For this review, take the finished solid that the model builds, in its own axes (mm). Face numbers are marked on the shaded views. A direction names the side the tool comes from. Round coordinates to 2 decimals unless told otherwise and drop trailing zeros. Order: outer loops, then holes, each group sorted by start corner. A loop starts at its lowest first (then second) coordinate and runs counter-clockwise, first axis right, second up. Notation, with made-up numbers: M 72.5,35.5 L 96.5,35.5 A26 ccw 96.5,62.5 Z; hole C 65.25,75 d5. An arc over 180 degrees is marked long. Use a Markdown table: item, result.
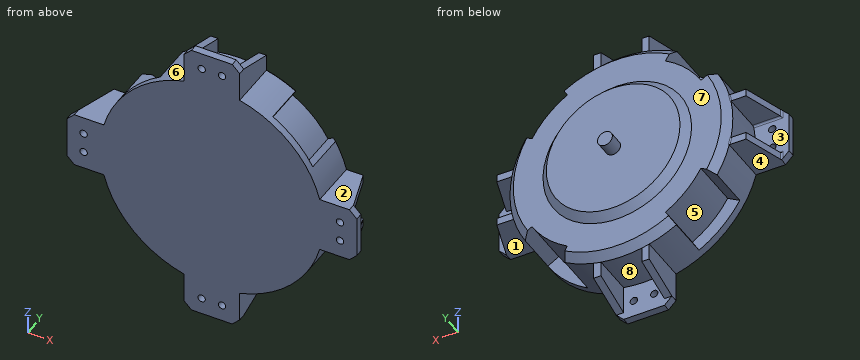
from build123d import *

# Parameters (mm, degrees)
SKETCH1_R                    = 150
BOSS_EXTRUDE1_DEPTH          = 75
CHAMFER1_SIZE                = 10
BOSS_EXTRUDE2_START          = -75
BOSS_EXTRUDE2_DEPTH          = 10
CHAMFER2_SIZE                = 10
BOSS_EXTRUDE3_DEPTH          = 10
SKETCH4_R                    = 5
CUT_EXTRUDE1_DEPTH           = 10
FILLET1_R                    = 2.5
FILLET2_R                    = 2.5
FILLET3_R                    = 2.5
CIRPATTERN4_COUNT            = 4
CIRPATTERN4_COPY_1_DEPTH     = 10
CIRPATTERN4_COPY_2_DEPTH     = 10
CIRPATTERN4_COPY_3_DEPTH     = 10
CIRPATTERN4_COPY_4_SKETCH_R  = 5
CIRPATTERN4_COPY_4_DEPTH     = 10
CIRPATTERN4_COPY_5_SKETCH_R  = 5
CIRPATTERN4_COPY_5_DEPTH     = 10
CIRPATTERN4_COPY_6_SKETCH_R  = 5
CIRPATTERN4_COPY_6_DEPTH     = 10
CHAMFER2_OF_CIRPATTERN4_SIZE = 10
CUT_EXTRUDE2_START           = -65
CUT_EXTRUDE2_DEPTH           = 65
CIRPATTERN5_COUNT            = 4
SKETCH6_R                    = 100
BOSS_EXTRUDE4_DEPTH          = 10
CHAMFER3_SIZE                = 10
SKETCH7_R                    = 10
BOSS_EXTRUDE5_DEPTH          = 20


# Some blends are built 0.0001 mm under size
with BuildPart() as part:
    # Sketch1 → Boss-Extrude1 (new body)
    with BuildSketch(Plane(origin=(0, 0, 0), x_dir=(1, 0, 0), z_dir=(0, 1, 0))):
        with Locations(Location((0, 0, 0), (0, 0, 270))):
            Circle(SKETCH1_R)
    extrude(amount=BOSS_EXTRUDE1_DEPTH)

    # Chamfer1
    chamfer1_edges = [part.edges().sort_by_distance(p)[0] for p in [
        (0, 75, -150),
    ]]
    chamfer(chamfer1_edges, length=CHAMFER1_SIZE)

    # Sketch2 → Boss-Extrude2 (add)
    with BuildSketch(Plane(origin=(0, 75, 0), x_dir=(1, 0, 0), z_dir=(0, 1, 0)).offset(BOSS_EXTRUDE2_START)):
        with BuildLine():
            Line((-195.236875483, -37.5), (-195.236875483, 37.5))
            Line((-195.236875483, 37.5), (-145.236875483, 37.5))
            ThreePointArc((-145.236875483, 37.5), (-150, 0), (-145.236875483, -37.5))
            Line((-145.236875483, -37.5), (-195.236875483, -37.5))
        make_face()
    boss_extrude2 = extrude(amount=BOSS_EXTRUDE2_DEPTH)

    # Chamfer2
    chamfer2_edges = [part.edges().sort_by_distance(p)[0] for p in [
        (-195.236875483, 5, -37.5),
        (-195.236875483, 5, 37.5),
    ]]
    chamfer(chamfer2_edges, length=CHAMFER2_SIZE)

    # Sketch3 → Boss-Extrude3 (add)
    with BuildSketch(Plane.XY.offset(37.5)):
        Polygon((-145.236875483, 0), (-145.236875483, 65), (-167.736875483, 65), (-185.236875483, 10), (-185.236875483, 0), align=None)
    boss_extrude3 = extrude(amount=-BOSS_EXTRUDE3_DEPTH)

    # Sketch4 → Cut-Extrude1 (cut)
    with BuildSketch(Plane(origin=(0, 10, 0), x_dir=(1, 0, 0), z_dir=(0, 1, 0))):
        with Locations(Location((-172.618437741, -13.75, 0), (0, 0, 270))):
            Circle(SKETCH4_R)
    cut_extrude1 = extrude(amount=-CUT_EXTRUDE1_DEPTH, mode=Mode.SUBTRACT)

    # Mirror2: Boss-Extrude3, Cut-Extrude1 across plane
    add(boss_extrude3.mirror(Plane(origin=(0, 0, 0), x_dir=(1, 0, 0), z_dir=(0, 0, -1))))
    add(cut_extrude1.mirror(Plane(origin=(0, 0, 0), x_dir=(1, 0, 0), z_dir=(0, 0, -1))), mode=Mode.SUBTRACT)

    # Fillet1
    fillet1_edges = [part.edges().sort_by_distance(p)[0] for p in [
        (-166.347248257, 10, -27.5),
        (-185.236875483, 10, -32.5),
    ]]
    fillet(fillet1_edges, radius=FILLET1_R)

    # Fillet2
    fillet2_edges = [part.edges().sort_by_distance(p)[0] for p in [
        (-166.347248257, 10, 27.5),
        (-185.236875483, 10, 32.5),
    ]]
    fillet(fillet2_edges, radius=FILLET2_R)

    # Fillet3
    # the kernel refuses this fillet: 2.5 mm, written as the material it adds along each edge
    with BuildSketch(Plane(origin=(0, 65, 0), x_dir=(-0.9860683765202287, 0, 0.1663404846294499), z_dir=(-0.1663404846294499, 0, -0.9860683765202287))) as fillet3_piece_1_section:
        with BuildLine():
            CenterArc((150 + FILLET3_R * 0.414213562373, FILLET3_R), FILLET3_R, 225, 45)
            Line((150 + FILLET3_R * 0.414213562373, 0), (150, 0))
            Line((150, 0), (150 - FILLET3_R * 0.292893218813, FILLET3_R * 0.292893218813))
        make_face()
    fillet3_piece_1 = revolve(axis=Axis((0, 65, 0), (0, 1, 0)), revolution_arc=5.891260177, mode=Mode.PRIVATE)
    fillet3_piece_1 = split(fillet3_piece_1, bisect_by=Plane(origin=(-146.208853891, 65.259294833, 27.5), z_dir=(0, 0, 1)), keep=Keep.TOP, mode=Mode.PRIVATE)
    fillet3_piece_1 = split(fillet3_piece_1, bisect_by=Plane(origin=(-146.208853891, 65.259294833, 37.5), z_dir=(0, 0, -1)), keep=Keep.TOP, mode=Mode.PRIVATE)
    add(fillet3_piece_1)
    with BuildSketch(Plane(origin=(0, 65, 0), x_dir=(-0.9637871207414556, 0, -0.2666728068118214), z_dir=(0.2666728068118214, 0, -0.9637871207414556))) as fillet3_piece_2_section:
        with BuildLine():
            CenterArc((150 + FILLET3_R * 0.414213562373, FILLET3_R), FILLET3_R, 225, 45)
            Line((150 + FILLET3_R * 0.414213562373, 0), (150, 0))
            Line((150, 0), (150 - FILLET3_R * 0.292893218813, FILLET3_R * 0.292893218813))
        make_face()
    fillet3_piece_2 = revolve(axis=Axis((0, 65, 0), (0, 1, 0)), revolution_arc=5.891260177, mode=Mode.PRIVATE)
    fillet3_piece_2 = split(fillet3_piece_2, bisect_by=Plane(origin=(-146.20885389, 65.259294833, -27.5), z_dir=(0, 0, -1)), keep=Keep.TOP, mode=Mode.PRIVATE)
    fillet3_piece_2 = split(fillet3_piece_2, bisect_by=Plane(origin=(-146.20885389, 65.259294833, -37.5), z_dir=(0, 0, 1)), keep=Keep.TOP, mode=Mode.PRIVATE)
    add(fillet3_piece_2)

    # CirPattern4: Boss-Extrude2, Boss-Extrude3, Cut-Extrude1 ×4 about axis
    cirpattern4_axis = Axis((0, 0, 0), (0, 1, 0))
    add([boss_extrude2.rotate(cirpattern4_axis, i * 360 / CIRPATTERN4_COUNT) for i in range(1, CIRPATTERN4_COUNT)])
    add([boss_extrude3.rotate(cirpattern4_axis, i * 360 / CIRPATTERN4_COUNT) for i in range(1, CIRPATTERN4_COUNT)])
    add([cut_extrude1.rotate(cirpattern4_axis, i * 360 / CIRPATTERN4_COUNT) for i in range(1, CIRPATTERN4_COUNT)], mode=Mode.SUBTRACT)

    # CirPattern4 copy 1 sketch → CirPattern4 copy 1 (add)
    with BuildSketch(Plane(origin=(-37.5, 0, 0), x_dir=(0, 0, -1), z_dir=(-1, 0, 0))):
        Polygon((-145.236875483, 0), (-145.236875483, -65), (-167.736875483, -65), (-185.236875483, -10), (-185.236875483, 0), align=None)
    extrude(amount=-CIRPATTERN4_COPY_1_DEPTH)

    # CirPattern4 copy 2 sketch → CirPattern4 copy 2 (add)
    with BuildSketch(Plane(origin=(0, 0, 37.5), x_dir=(-1, 0, 0), z_dir=(0, 0, 1))):
        Polygon((-145.236875483, 0), (-145.236875483, -65), (-167.736875483, -65), (-185.236875483, -10), (-185.236875483, 0), align=None)
    extrude(amount=-CIRPATTERN4_COPY_2_DEPTH)

    # CirPattern4 copy 3 sketch → CirPattern4 copy 3 (add)
    with BuildSketch(Plane(origin=(37.5, 0, 0), x_dir=(0, 0, 1), z_dir=(1, 0, 0))):
        Polygon((-145.236875483, 0), (-145.236875483, -65), (-167.736875483, -65), (-185.236875483, -10), (-185.236875483, 0), align=None)
    extrude(amount=-CIRPATTERN4_COPY_3_DEPTH)

    # CirPattern4 copy 4 sketch → CirPattern4 copy 4 (cut)
    with BuildSketch(Plane(origin=(0, 10, 0), x_dir=(0, 0, -1), z_dir=(0, 1, 0))):
        with Locations((-172.618437741, 13.75)):
            Circle(CIRPATTERN4_COPY_4_SKETCH_R)
    extrude(amount=-CIRPATTERN4_COPY_4_DEPTH, mode=Mode.SUBTRACT)

    # CirPattern4 copy 5 sketch → CirPattern4 copy 5 (cut)
    with BuildSketch(Plane(origin=(0, 10, 0), x_dir=(-1, 0, 0), z_dir=(0, 1, 0))):
        with Locations((-172.618437741, 13.75)):
            Circle(CIRPATTERN4_COPY_5_SKETCH_R)
    extrude(amount=-CIRPATTERN4_COPY_5_DEPTH, mode=Mode.SUBTRACT)

    # CirPattern4 copy 6 sketch → CirPattern4 copy 6 (cut)
    with BuildSketch(Plane.ZX.offset(10)):
        with Locations((-172.618437741, 13.75)):
            Circle(CIRPATTERN4_COPY_6_SKETCH_R)
    extrude(amount=-CIRPATTERN4_COPY_6_DEPTH, mode=Mode.SUBTRACT)

    # Chamfer2 of CirPattern4
    chamfer2_of_cirpattern4_edges = [part.edges().sort_by_distance(p)[0] for p in [
        (-37.5, 5, 195.236875483),
        (37.5, 5, 195.236875483),
        (195.236875483, 5, 37.5),
        (195.236875483, 5, -37.5),
        (37.5, 5, -195.236875483),
        (-37.5, 5, -195.236875483),
    ]]
    chamfer(chamfer2_of_cirpattern4_edges, length=CHAMFER2_OF_CIRPATTERN4_SIZE)

    # Sketch5 → Cut-Extrude2 (cut)
    with BuildSketch(Plane(origin=(0, 75, 0), x_dir=(1, 0, 0), z_dir=(0, 1, 0)).offset(CUT_EXTRUDE2_START)):
        with BuildLine():
            Line((-112.583302492, -65), (-129.903810568, -75))
            ThreePointArc((-129.903810568, -75), (-106.066017178, -106.066017178), (-75, -129.903810568))
            Line((-75, -129.903810568), (-65, -112.583302492))
            ThreePointArc((-65, -112.583302492), (-91.923881554, -91.923881554), (-112.583302492, -65))
        make_face()
    cut_extrude2 = extrude(amount=CUT_EXTRUDE2_DEPTH, mode=Mode.SUBTRACT)

    # CirPattern5: Cut-Extrude2 ×4 about axis
    cirpattern5_axis = Axis((1.096442134, 0, -1.096442134), (0, 1, 0))
    for i in range(1, CIRPATTERN5_COUNT):
        add(cut_extrude2.rotate(cirpattern5_axis, i * 360 / CIRPATTERN5_COUNT), mode=Mode.SUBTRACT)

    # Sketch6 → Boss-Extrude4 (add)
    with BuildSketch(Plane(origin=(0, 75, 0), x_dir=(1, 0, 0), z_dir=(0, 1, 0))):
        with Locations(Location((0, 0, 0), (0, 0, 270))):
            Circle(SKETCH6_R)
    extrude(amount=BOSS_EXTRUDE4_DEPTH)

    # Chamfer3
    chamfer3_edges = [part.edges().sort_by_distance(p)[0] for p in [
        (0, 85, -100),
    ]]
    chamfer(chamfer3_edges, length=CHAMFER3_SIZE - 0.0001)  # a hair under: the kernel refuses the full size

    # Sketch7 → Boss-Extrude5 (add)
    with BuildSketch(Plane(origin=(0, 85, 0), x_dir=(1, 0, 0), z_dir=(0, 1, 0))):
        with Locations(Location((0, 0, 0), (0, 0, 270))):
            Circle(SKETCH7_R)
    extrude(amount=BOSS_EXTRUDE5_DEPTH)


solid = part.part
Q1. Draft analysis for pull direction X (two halves, no side actions). For the marked faces 5, 6, 7 and 8, state which applies: pulls with the +X half, pulls with the -X half, needs draft (parallel to the pull), parting line crosses it, or undercut.
Determined:
| item | result |
|---|---|
| face 5 | undercut |
| face 6 | pulls with the -X half |
| face 7 | needs draft |
| face 8 | undercut |
Q2. Wall thickness on line 1 along X through (y, z) = (8, -13) (3 decimals); line 2 along Z through (x, y) = (-13.75, 2.75); line 3 along X through (y, z) = (28.5, -172.5): over which ranges is each line inside the solid? List them lowest first. Write a range as [from, to].
Determined:
| item | result |
|---|---|
| line 1 | x = [-195.237, -177.562], [-167.675, 167.675], [177.562, 195.237] |
| line 2 | z = [-195.24, -177.62], [-167.62, 167.62], [177.62, 195.24] |
| line 3 | x = [-37.5, -27.5], [27.5, 37.5] |
Q3. Add section A-A (z = 163). Write out the cut boundary in (x, y), then the cut area to 3 significant figures.
Determined:
| item | result |
|---|---|
| outline | M -37.5,0 L 37.5,0 L 37.5,65 L 27.5,65 L 27.5,10 L -27.5,10 L -27.5,65 L -37.5,65 Z |
| area | 1,850 mm^2 |
Q4. Machinability: for the marked faces 1, 2, 3 and 4, which of the approach directions +Z, -Z, +X, -X, +Y, -Y give a long, thin tool a straight path to every point of the face, cutting with its end or side? Answer none if there is none.
Determined:
| item | result |
|---|---|
| face 1 | -Z, +X, +Y, -Y |
| face 2 | +Z, +X, +Y, -Y |
| face 3 | -X, +Y |
| face 4 | -Z, -X, +Y, -Y |
Q5. Add section C-C (y = 91). Write out the cut boundary in (x, z).
Determined:
| item | result |
|---|---|
| outline | C 0,0 d20 |
Q6. Clearance check with flat-ended pins moving along their axes: pin 1 (1.5 mm diameter, centred on x = 122.5, y = 62, fed in from -Z); pin 2 (24 mm diameter, centred on x = -10, z = -163, fed in from +Y); pin 3 (20 mm diameter, centred on y = 19.5, z = 169, fed in from -X); pin 4 (12 mm diameter, centred on x = 139.5, y = 83.5, fed in from -Z). State where each tip first meets the part, or that it passes through.
Determined:
| item | result |
|---|---|
| pin 1 | stops at z = -72.09 |
| pin 2 | stops at y = 10 |
| pin 3 | stops at x = -37.5 |
| pin 4 | passes through |
